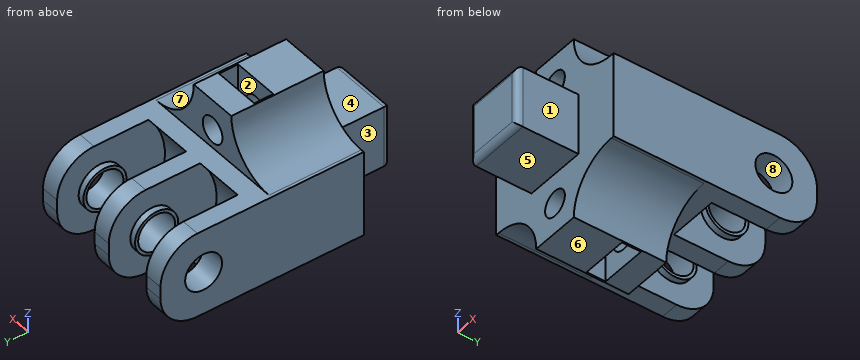
```python
from build123d import *

# Parameters (mm, degrees)
SKETCH_1_W               = 3
SKETCH_1_H               = 18
EXTRUDE_2_DEPTH          = 7
CUT_EXTRUDE_1_DEPTH      = 32.591137998
CUT_EXTRUDE_1_DEPTH_BACK = 7.591137998
CUT_EXTRUDE_1_START      = -25
SKETCH_3_R               = 3
SKETCH_15_R              = 3.5
SKETCH_15_R_2            = 3
EXTRUDE_11_DEPTH         = 1
EXTRUDE_START            = 1
SKETCH_5_R               = 3.5
SKETCH_5_R_2             = 3
EXTRUDE_6_DEPTH          = 1
SKETCH_6_R               = 3.5
SKETCH_6_R_2             = 3
EXTRUDE_7_DEPTH          = 1
SKETCH_7_R               = 3.5
SKETCH_7_R_2             = 3
EXTRUDE_8_DEPTH          = 1
FILLET_1_R               = 6
SKETCH_8_W               = 10
SKETCH_8_H               = 10
EXTRUDE_9_DEPTH          = 10
FILLET_2_R               = 1
EXTRUDE_START_2          = -22
EXTRUDE_14_DEPTH         = 19
SKETCH_17_W              = 8
SKETCH_17_H              = 8
SKETCH_17_R              = 2.1
EXTRUDE_12_DEPTH         = 8
EXTRUDE_START_3          = -7
SKETCH_17_2_W            = 8
SKETCH_17_2_H            = 8
SKETCH_17_2_R            = 2.1
EXTRUDE_13_DEPTH         = 7
CUT_EXTRUDE_2_DEPTH      = 3.1
FILLET_4_R               = 8


with BuildPart() as part:
    # 草图1 → 凸台-拉伸2 (new, symmetric)
    with BuildSketch(Plane.XY):
        Polygon((3, 0), (0, 0), (0, -15), (25, -15), (25, 0), (22, 0), (14, 0), (11, 0), align=None)
        with Locations((12.5, 9)):
            Rectangle(SKETCH_1_W, SKETCH_1_H)
        with Locations((23.5, 9)):
            Rectangle(SKETCH_1_W, SKETCH_1_H)
        with Locations((1.5, 9)):
            Rectangle(SKETCH_1_W, SKETCH_1_H)
    extrude(amount=EXTRUDE_2_DEPTH, both=True)

    # 草图3 → 切除-拉伸1 (cut, two sides: drawn at the far end of the back side and taken through both)
    with BuildSketch(Plane(origin=(25, 0, 0), x_dir=(0, 0, -1), z_dir=(1, 0, 0)).offset(CUT_EXTRUDE_1_START - CUT_EXTRUDE_1_DEPTH_BACK)):
        with Locations(Location((0, 11, 0), (0, 0, 90))):
            Circle(SKETCH_3_R)
    extrude(amount=CUT_EXTRUDE_1_DEPTH + CUT_EXTRUDE_1_DEPTH_BACK, mode=Mode.SUBTRACT)

    # 草图15 → 凸台-拉伸11 (add)
    with BuildSketch(Plane(origin=(3, 0, 0), x_dir=(0, 0, -1), z_dir=(1, 0, 0))):
        with Locations(Location((0, 11, 0), (0, 0, 180))):
            Circle(SKETCH_15_R)
        with Locations(Location((0, 11, 0), (0, 0, 90))):
            Circle(SKETCH_15_R_2, mode=Mode.SUBTRACT)
    extrude(amount=EXTRUDE_11_DEPTH)

    # 草图5 → 凸台-拉伸6 (add)
    with BuildSketch(Plane.ZY.offset(-11).offset(EXTRUDE_START)):
        with Locations((0, 11)):
            Circle(SKETCH_5_R)
        with Locations(Location((0, 11, 0), (0, 0, 90))):
            Circle(SKETCH_5_R_2, mode=Mode.SUBTRACT)
    extrude(amount=-EXTRUDE_6_DEPTH)

    # 草图6 → 凸台-拉伸7 (add)
    with BuildSketch(Plane(origin=(14, 0, 0), x_dir=(0, 0, -1), z_dir=(1, 0, 0))):
        with Locations(Location((0, 11, 0), (0, 0, 180))):
            Circle(SKETCH_6_R)
        with Locations(Location((0, 11, 0), (0, 0, 90))):
            Circle(SKETCH_6_R_2, mode=Mode.SUBTRACT)
    extrude(amount=EXTRUDE_7_DEPTH)

    # 草图7 → 凸台-拉伸8 (add)
    with BuildSketch(Plane.ZY.offset(-22).offset(EXTRUDE_START)):
        with Locations((0, 11)):
            Circle(SKETCH_7_R)
        with Locations(Location((0, 11, 0), (0, 0, 90))):
            Circle(SKETCH_7_R_2, mode=Mode.SUBTRACT)
    extrude(amount=-EXTRUDE_8_DEPTH)

    # 圆角1
    fillet_1_edges = [part.edges().sort_by_distance(p)[0] for p in [
        (23.5, 18, 7),
        (1.5, 18, -7),
        (12.5, 18, -7),
        (23.5, 18, -7),
        (12.5, 18, 7),
        (1.5, 18, 7),
    ]]
    fillet(fillet_1_edges, radius=FILLET_1_R)

    # 草图8 → 凸台-拉伸9 (add)
    with BuildSketch(Plane.XZ.offset(15)):
        with Locations((12.5, 0)):
            Rectangle(SKETCH_8_W, SKETCH_8_H)
    extrude(amount=EXTRUDE_9_DEPTH)

    # 圆角2
    fillet_2_edges = [part.edges().sort_by_distance(p)[0] for p in [
        (12.5, -25, 5),
        (7.5, -25, 0),
        (12.5, -25, -5),
        (17.5, -25, 0),
    ]]
    fillet(fillet_2_edges, radius=FILLET_2_R)

    # 草图23 → 凸台-拉伸14 (add)
    with BuildSketch(Plane.ZY.offset(EXTRUDE_START_2)):
        with BuildLine():
            Line((-7, -7), (7, -7))
            Line((7, -7), (7, 3.173762079))
            ThreePointArc((7, 3.173762079), (0, 0.5), (-7, 3.173762079))
            Line((-7, 3.173762079), (-7, -7))
        make_face()
    extrude(amount=EXTRUDE_14_DEPTH)

    # 草图17 → 凸台-拉伸12 (add)
    with BuildSketch(Plane(origin=(0, -7, 0), x_dir=(-1, 0, 0), z_dir=(0, -1, 0))):
        with Locations((-12.51246086, 11)):
            Rectangle(SKETCH_17_W, SKETCH_17_H)
        with Locations(Location((-12.5, 10, 0), (0, 0, 270))):
            Circle(SKETCH_17_R, mode=Mode.SUBTRACT)
    extrude_12 = extrude(amount=EXTRUDE_12_DEPTH)

    # 草图17<2> → 凸台-拉伸13 (add)
    with BuildSketch(Plane(origin=(0, -7, 0), x_dir=(-1, 0, 0), z_dir=(0, -1, 0)).offset(EXTRUDE_START_3)):
        with Locations((-12.51246086, 11)):
            Rectangle(SKETCH_17_2_W, SKETCH_17_2_H)
        with Locations(Location((-12.5, 10, 0), (0, 0, 270))):
            Circle(SKETCH_17_2_R, mode=Mode.SUBTRACT)
    extrude_13 = extrude(amount=EXTRUDE_13_DEPTH)

    # 草图18 → 切除-拉伸2 (cut)
    with BuildSketch(Plane(origin=(0, -7, 0), x_dir=(-1, 0, 0), z_dir=(0, -1, 0))):
        Polygon((-8.75, 15), (-8.75, 12.165063509), (-12.5, 14.330127019), (-16.25, 12.165063509), (-16.25, 15), align=None)
        Polygon((-8.75, 7.834936491), (-8.75, 12.165063509), (-12.5, 14.330127019), (-16.25, 12.165063509), (-16.25, 7.834936491), (-12.5, 5.669872981), align=None)
    cut_extrude_2 = extrude(amount=-CUT_EXTRUDE_2_DEPTH, mode=Mode.SUBTRACT)

    # 镜向1: 凸台-拉伸12, 凸台-拉伸13, 切除-拉伸2 across plane
    add(extrude_12.mirror(Plane.XY))
    add(extrude_13.mirror(Plane.XY))
    add(cut_extrude_2.mirror(Plane.XY), mode=Mode.SUBTRACT)

    # 圆角4
    fillet_4_edges = [part.edges().sort_by_distance(p)[0] for p in [
        (8.51246086, -7.5, -7),
        (16.51246086, -7.5, -7),
        (16.51246086, -7.5, 7),
        (8.51246086, -7.5, 7),
    ]]
    fillet(fillet_4_edges, radius=FILLET_4_R - 0.0001)  # a hair under: the kernel refuses the full size


solid = part.part
```
Verification items for the finished model (mm, model axes). Face numbers are marked on the shaded views. A direction names the side the tool comes from. Round coordinates to 2 decimals unless told otherwise and drop trailing zeros. Write each loop counter-clockwise with the first axis right and the second up, starting at its lowest first coordinate (ties: lowest second). Pieces come first, ordered by that corner, then holes. Notation, with made-up numbers: (88.5, -17) -> (139.5, -17) arc R21 cw to (139.5, 11) -> close; hole circle Ø9 at (26, 11). An arc over 180 degrees is marked (long way). Write each question's results on one line, items separated by ' | '. Start each with the question number.
1. Set-up check for the marked faces 1, 2, 3, 4 and 5: record each of +Z, -Z, +X, -X, +Y, -Y from which the full face is reachable in a straight line by a thin tool's end or side.
2. Cross-section at B-B (y = 15). Enter the section's corners in (x, z).
3. Material ranges on probe 1 along Z at (x, y) = (12.5, -2.2); probe 2 along X at (y, z) = (14, 1.25); probe 3 along Z at (x, y) = (22.7, 11), recorded low to high. Write a range as from..to.
4. Cross-section at D-D (z = 6.5). Enter the section's corners in (x, y).
5. Draft check along Z on the marked faces 6, 7 and 8. Enter one of: +Z half, -Z half, draft (parallel to the pull), parting line (faces both ways), or undercut.
6. Cross-section at A-A (y = -3). Count the separate pieces of the cut face and the enclosed holes in it, then the cut area to 3 significant figures.
7. Depth check by flat-ended pin: P1, Ø2, axis at x = 14.5, z = -9.5, coming from the +Y side; P2, Ø4, axis at x = 12, z = -11, coming from the -Y side; P3, Ø2, axis at x = 5.5, y = -4.5, coming from the -Z side. Enter the tip coordinate at first touch or a pass-through.
8. Cross-section at C-C (z = -10). Enter the section's corners in (x, y), then the cut area to 3 significant figures.
Solutions:
1) face 1: +Z, -Z, +X, -Y | face 2: +Z | face 3: +Z, -Z, -X, -Y | face 4: +Z, +X, -X, -Y | face 5: -Z, +X, -X, -Y
2) outline: (0, -6.2) -> (3, -6.2) -> (3, 6.2) -> (0, 6.2) -> close; (11, -6.2) -> (14, -6.2) -> (14, 6.2) -> (11, 6.2) -> close; (22, -6.2) -> (25, -6.2) -> (25, 6.2) -> (22, 6.2) -> close
3) probe 1: z = -15..-12.1, -7.9..7.9, 12.1..15 | probe 2: x = 0..4, 10..15, 21..25 | probe 3: z = -7..-3, 3..7
4) outline: (0, -15) -> (25, -15) -> (25, 14.4) -> (22, 14.4) -> (22, 2.75) -> (14, 2.75) -> (14, 14.4) -> (11, 14.4) -> (11, 2.75) -> (3, 2.75) -> (3, 14.4) -> (0, 14.4) -> close; hole (11.06, -7) -> (13.94, -7) -> (13.94, -3.9) -> (11.06, -3.9) -> close
5) face 6: -Z half | face 7: +Z half | face 8: undercut
6) separate pieces: 1 | enclosed holes: 2 | area: 505 mm2
7) P1: stops at y = 0 | P2: stops at y = -15 | P3: stops at z = -9.69
8) outline: (6.76, -15) -> (10.4, -15) -> (10.4, -7) -> (8.75, -7) -> (8.75, -3.9) -> (10.4, -3.9) -> (10.4, 0) -> (6.76, 0) -> close; (14.6, -15) -> (18.27, -15) -> (18.27, 0) -> (14.6, 0) -> (14.6, -3.9) -> (16.25, -3.9) -> (16.25, -7) -> (14.6, -7) -> close | area: 99.4 mm2
